```python
from build123d import *

# Parameters (mm, degrees)
BOSS_EXTRUDE1_DEPTH = 3.25


with BuildPart() as part:
    # Sketch1 → Boss-Extrude1 (new body)
    with BuildSketch(Plane.XY):
        with BuildLine():
            ThreePointArc((44.089679783, 33.952554996), (51.06531213, 24.285160039), (55.70378497, 13.303241189))
            Line((55.70378497, 13.303241189), (103.739324528, 13.303241189))
            ThreePointArc((103.739324528, 13.303241189), (4.870724861, 98.303241189), (-93.997874805, 13.303241189))
            Line((-93.997874805, 13.303241189), (-45.962335247, 13.303241189))
            ThreePointArc((-45.962335247, 13.303241189), (-41.323862407, 24.285160039), (-34.34823006, 33.952554996))
            ThreePointArc((-34.34823006, 33.952554996), (-27.759333331, 40.067811131), (-20.231728052, 44.981575111))
            ThreePointArc((-20.231728052, 44.981575111), (-13.256342735, 48.106950091), (-5.903935262, 50.19646521))
            ThreePointArc((-5.903935262, 50.19646521), (4.870724861, 51.303241189), (15.645384984, 50.19646521))
            ThreePointArc((15.645384984, 50.19646521), (22.997792458, 48.106950091), (29.973177775, 44.981575111))
            ThreePointArc((29.973177775, 44.981575111), (37.500783054, 40.067811131), (44.089679783, 33.952554996))
        make_face()
        with BuildLine():
            Line((103.739324528, 13.303241189), (55.70378497, 13.303241189))
            ThreePointArc((55.70378497, 13.303241189), (57.326192573, 5.881097557), (57.870724861, -1.696758811))
            ThreePointArc((57.870724861, -1.696758811), (57.326192573, -9.274615178), (55.70378497, -16.696758811))
            Line((55.70378497, -16.696758811), (103.739324528, -16.696758811))
            ThreePointArc((103.739324528, -16.696758811), (104.587473622, -9.218062998), (104.870724861, -1.696758811))
            ThreePointArc((104.870724861, -1.696758811), (104.587473622, 5.824545377), (103.739324528, 13.303241189))
        make_face()
        with BuildLine():
            ThreePointArc((-45.962335247, -16.696758811), (-48.129275139, -1.696758811), (-45.962335247, 13.303241189))
            Line((-45.962335247, 13.303241189), (-93.997874805, 13.303241189))
            ThreePointArc((-93.997874805, 13.303241189), (-95.129275139, -1.696758811), (-93.997874805, -16.696758811))
            Line((-93.997874805, -16.696758811), (-45.962335247, -16.696758811))
        make_face()
        with BuildLine():
            Line((52.514618421, 13.303241189), (36.493501463, 13.303241189))
            ThreePointArc((36.493501463, 13.303241189), (39.01598208, 5.990985297), (39.870724861, -1.696758811))
            ThreePointArc((39.870724861, -1.696758811), (39.01598208, -9.384502919), (36.493501463, -16.696758811))
            Line((36.493501463, -16.696758811), (52.514618421, -16.696758811))
            ThreePointArc((52.514618421, -16.696758811), (54.24036914, -9.284829533), (54.820105173, -1.696758811))
            ThreePointArc((54.820105173, -1.696758811), (54.24036914, 5.891311912), (52.514618421, 13.303241189))
        make_face()
        with BuildLine():
            ThreePointArc((-26.75205174, -16.696758811), (-30.129275139, -1.696758811), (-26.75205174, 13.303241189))
            Line((-26.75205174, 13.303241189), (-42.773168698, 13.303241189))
            ThreePointArc((-42.773168698, 13.303241189), (-45.07865545, -1.696758811), (-42.773168698, -16.696758811))
            Line((-42.773168698, -16.696758811), (-26.75205174, -16.696758811))
        make_face()
        with BuildLine():
            Line((55.70378497, 13.303241189), (52.514618421, 13.303241189))
            ThreePointArc((52.514618421, 13.303241189), (54.24036914, 5.891311912), (54.820105173, -1.696758811))
            ThreePointArc((54.820105173, -1.696758811), (54.24036914, -9.284829533), (52.514618421, -16.696758811))
            Line((52.514618421, -16.696758811), (55.70378497, -16.696758811))
            ThreePointArc((55.70378497, -16.696758811), (57.326192573, -9.274615178), (57.870724861, -1.696758811))
            ThreePointArc((57.870724861, -1.696758811), (57.326192573, 5.881097557), (55.70378497, 13.303241189))
        make_face()
        with BuildLine():
            ThreePointArc((-42.773168698, -16.696758811), (-45.07865545, -1.696758811), (-42.773168698, 13.303241189))
            Line((-42.773168698, 13.303241189), (-45.962335247, 13.303241189))
            ThreePointArc((-45.962335247, 13.303241189), (-48.129275139, -1.696758811), (-45.962335247, -16.696758811))
            Line((-45.962335247, -16.696758811), (-42.773168698, -16.696758811))
        make_face()
        with BuildLine():
            ThreePointArc((39.870724861, -1.696758811), (39.01598208, 5.990985297), (36.493501463, 13.303241189))
            Line((36.493501463, 13.303241189), (-26.75205174, 13.303241189))
            ThreePointArc((-26.75205174, 13.303241189), (-30.129275139, -1.696758811), (-26.75205174, -16.696758811))
            Line((-26.75205174, -16.696758811), (36.493501463, -16.696758811))
            ThreePointArc((36.493501463, -16.696758811), (39.01598208, -9.384502919), (39.870724861, -1.696758811))
        make_face()
        with BuildLine():
            ThreePointArc((-34.34823006, -37.346072617), (-41.323862407, -27.67867766), (-45.962335247, -16.696758811))
            Line((-45.962335247, -16.696758811), (-93.997874805, -16.696758811))
            ThreePointArc((-93.997874805, -16.696758811), (4.870724861, -101.696758811), (103.739324528, -16.696758811))
            Line((103.739324528, -16.696758811), (55.70378497, -16.696758811))
            ThreePointArc((55.70378497, -16.696758811), (51.06531213, -27.67867766), (44.089679783, -37.346072617))
            ThreePointArc((44.089679783, -37.346072617), (38.582870536, -42.59286173), (32.381730977, -46.997360821))
            ThreePointArc((32.381730977, -46.997360821), (4.870724861, -54.696758811), (-22.640281254, -46.997360821))
            ThreePointArc((-22.640281254, -46.997360821), (-28.841420813, -42.59286173), (-34.34823006, -37.346072617))
        make_face()
    extrude(amount=BOSS_EXTRUDE1_DEPTH)


solid = part.part
```
Verification items for the finished model (mm, model axes). Coordinates: 2 decimals unless noted, no trailing zeros. Loops run counter-clockwise (first coordinate to the right, second up) from the corner with the lowest first, then second, coordinate; pieces in that order, holes last. Notation, with made-up numbers: (67.5, 0.25) -> (73.5, 0.25) arc R29 cw to (73.5, 27.25) -> close; hole circle Ø9 at (61, -16.5). An arc over 180 degrees is marked (long way). Answer in a Markdown table with one row per item.
1) Section check B-B (y = -25.5). Record the cut outline in (x, z) (3 decimals).
The answers:
| item | result |
|---|---|
| outline | (-92.255, 0) -> (-42.483, 0) -> (-42.483, 3.25) -> (-92.255, 3.25) -> close; (52.225, 0) -> (101.996, 0) -> (101.996, 3.25) -> (52.225, 3.25) -> close |
2) Scan lines: line 1 along Y through (x, z) = (4.5, 2.2); line 2 along Y through (x, z) = (-31, 2.7); line 3 along X through (y, z) = (-43.5, 1.6). Record each from-to range of solid material in increasing order. Write a range as from..to.
The answers:
| item | result |
|---|---|
| line 1 | y = -101.7..-54.7, -16.7..13.3, 51.3..98.3 |
| line 2 | y = -95.04..-40.71, -16.7..13.3, 37.32..91.65 |
| line 3 | x = -85.97..-27.71, 37.45..95.71 |
3) Depth check by flat-ended pin: P1, Ø1.5, axis at x = -13, z = 0.5, coming from the +Y side; P2, Ø1, axis at x = 78.5, z = 1, coming from the -Y side; P3, Ø1.6, axis at x = 3.5, z = 1, coming from the +Y side. Enter the tip coordinate at first touch or a pass-through.
The answers:
| item | result |
|---|---|
| P1 | stops at y = 96.83 |
| P2 | stops at y = -69.9 |
| P3 | stops at y = 98.3 |
4) Section check D-D (y = 27). Record the cut outline in (x, z).
The answers:
| item | result |
|---|---|
| outline | (-90.92, 0) -> (-39.69, 0) -> (-39.69, 3.25) -> (-90.92, 3.25) -> close; (49.43, 0) -> (100.66, 0) -> (100.66, 3.25) -> (49.43, 3.25) -> close |
5) Section check C-C (x = -2). Record the cut outline in (y, z).
The answers:
| item | result |
|---|---|
| outline | (-101.46, 0) -> (-54.25, 0) -> (-54.25, 3.25) -> (-101.46, 3.25) -> close; (-16.7, 0) -> (13.3, 0) -> (13.3, 3.25) -> (-16.7, 3.25) -> close; (50.86, 0) -> (98.07, 0) -> (98.07, 3.25) -> (50.86, 3.25) -> close |
6) Section check A-A (z = 2.5). Record the cut outline in (x, y), and give its area (3 significant figures).
The answers:
| item | result |
|---|---|
| outline | circle Ø200 at (4.87, -1.7); hole (-45.96, -16.7) arc R53 ccw to (55.7, -16.7) -> close; hole (-45.96, 13.3) -> (55.7, 13.3) arc R53 ccw to start |
| area | 25,700 mm2 |
